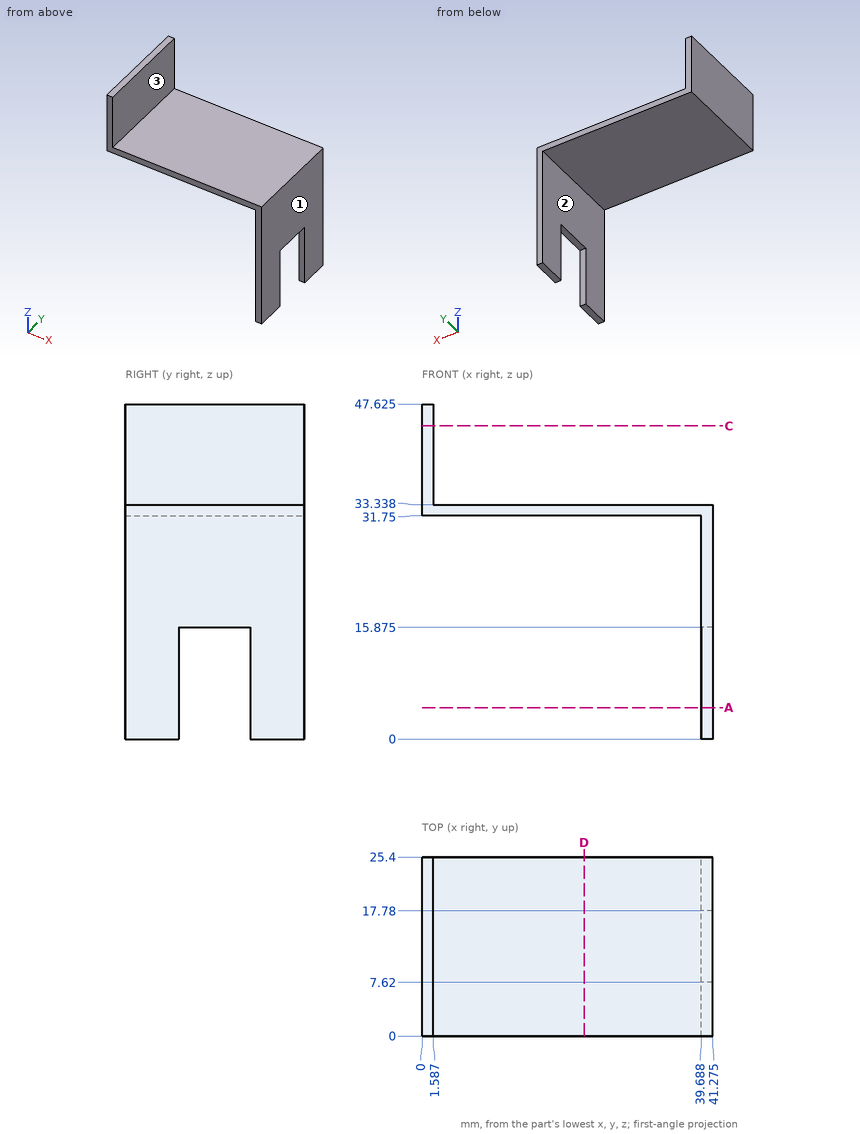
Source: three-view drawing plus pictorial views. Frame: mm from the lowest corner of the part. A direction names the side the tool comes from. Round coordinates to 2 decimals unless told otherwise and drop trailing zeros. Loops run counter-clockwise (first coordinate to the right, second up) from the corner with the lowest first, then second, coordinate; pieces in that order, holes last.
1. Ray query, L1, parallel to Z at x = 16, y = 20.25; L2, parallel to X at y = 16.75, z = 45; L3, parallel to X at y = 20, z = 29 (1 decimal). Return the intervals inside material, ascending.
2. Section query A-A on z = 4.5. Output: boundary loops of the cut face in (x, y) (1 decimal), and give its area (3 significant figures).
3. Section query C-C on z = 44.5. Output: boundary loops of the cut face in (x, y).
4. Access query for the marked faces 1, 2 and 3. Directions: +Z, -Z, +X, -X, +Y, -Y. A direction counts if a zero-diameter tool reaches every point of the face in a straight line with its end or side. Return the directions, or none.
5. Section query D-D on x = 23. Output: boundary loops of the cut face in (y, z).
6. Contact query for flat-ended pins moving along their axis: pin 1 (5 mm diameter, centred on x = 29.5, y = 15, fed in from -Z); pin 2 (2 mm diameter, centred on x = 5, y = 4, fed in from +Z); pin 3 (12.5 mm diameter, centred on y = 17.5, z = 16.5, fed in from -X); pin 4 (0.5 mm diameter, centred on x = 41, z = 7, fed in from -Y). Output: stop coordinate, or through.
Answers below:
1. L1: z = 31.75 to 33.34
1. L2: x = 0 to 1.59
1. L3: x = 39.7 to 41.3
2. outline: (39.7, 0) - (41.3, 0) - (41.3, 7.6) - (39.7, 7.6) - close; (39.7, 17.8) - (41.3, 17.8) - (41.3, 25.4) - (39.7, 25.4) - close
2. area: 24.2 mm2
3. outline: (0, 0) - (1.59, 0) - (1.59, 25.4) - (0, 25.4) - close
4. face 1: +Z, -Z, +X, +Y, -Y
4. face 2: -Z, -X, +Y, -Y
4. face 3: +Z, +X, +Y, -Y
5. outline: (0, 31.75) - (25.4, 31.75) - (25.4, 33.34) - (0, 33.34) - close
6. pin 1: stops at z = 31.75
6. pin 2: stops at z = 33.34
6. pin 3: stops at x = 39.69
6. pin 4: stops at y = 0
